The listing builds one solid part. Answer for the finished solid, in the listing's coordinates (mm). Face numbers are marked on the shaded views. A direction names the side the tool comes from. Give positions to 0.01 mm unless a question says otherwise; leave off trailing zeros. Write each loop counter-clockwise with the first axis right and the second up, starting at its lowest first coordinate (ties: lowest second). Pieces come first, ordered by that corner, then holes. Notation, with made-up numbers: (69, 54) - (106, 54) arc R31 cw to (106, 79) - close; hole circle Ø9 at (-18.5, -32.75). An arc over 180 degrees is marked (long way). One line per question, with ' | ' between items. Start each with the question number.
1. The mould has two halves that part along X. Classify the marked faces 5, 6, 7 and 8: +X half, -X half, draft (parallel to the pull), parting line (faces both ways), or undercut.
2. For the marked faces 1, 2, 3 and 4, determine the directions among +Z, -Z, +X, -X, +Y, -Y from which every point of the face is accessible in a straight line to the end or side of a thin tool.
3. A cutting plane is placed at A-A (z = 25). Determine the outline of the cut face in (x, y).
4. Given P1, Ø2, axis at y = 6.5, z = -7.5, coming from the -X side; P2, Ø10, axis at x = 1.5, y = 9.5, coming from the -Z side; P3, Ø10, axis at y = 6, z = -20.5, coming from the -X side; P4, Ø6, axis at x = -1.3, z = 25, coming from the -Y side, each flat-ended and moving along its own axis, determine where each tip first touches the part or whether it passes through.
5. A cutting plane is placed at D-D (z = 14.5). Determine the outline of the cut face in (x, y), then the cut area to 3 significant figures.
6. A cutting plane is placed at B-B (y = 14.5). Determine the outline of the cut face in (x, z), then the cut area to 3 significant figures.
7. Find the intervals of material crossed by L1, parallel to X at y = 9, z = 25; L2, parallel to X at y = 4.75, z = 37; L3, parallel to X at y = 12.25, z = -10, in increasing order. Write a range as from..to.
8. A cutting plane is placed at C-C (x = -13). Determine the outline of the cut face in (y, z).
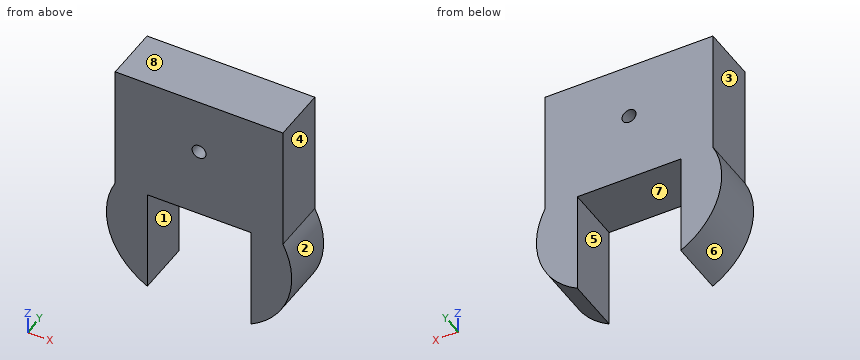
```python
from build123d import *

# Parameters (mm, degrees)
BOSS_EXTRUDE1_DEPTH = 20
SKETCH2_R           = 2.5
CUT_EXTRUDE1_DEPTH  = 20


with BuildPart() as part:
    # Sketch1 → Boss-Extrude1 (new body)
    with BuildSketch(Plane(origin=(0, 0, 0), x_dir=(1, 0, 0), z_dir=(0, 1, 0))):
        with BuildLine():
            Line((-19.801702617, 0), (17.198297383, 0))
            Line((17.198297383, 0), (17.198297383, 37))
            ThreePointArc((17.198297383, 37), (30.611248287, 20.881727984), (28.698297383, 0))
            Line((28.698297383, 0), (28.698297383, -45))
            Line((28.698297383, -45), (-31.301702617, -45))
            Line((-31.301702617, -45), (-31.301702617, 0))
            ThreePointArc((-31.301702617, 0), (-33.214653521, 20.881727984), (-19.801702617, 37))
            Line((-19.801702617, 37), (-19.801702617, 0))
        make_face()
    extrude(amount=BOSS_EXTRUDE1_DEPTH)

    # Sketch2 → Cut-Extrude1 (cut)
    with BuildSketch(Plane(origin=(0, 20, 0), x_dir=(1, 0, 0), z_dir=(0, 1, 0))):
        with Locations(Location((-1.301702617, -25, 0), (0, 0, 270))):
            Circle(SKETCH2_R)
    extrude(amount=-CUT_EXTRUDE1_DEPTH, mode=Mode.SUBTRACT)


solid = part.part
```
Determined:
1) face 5: undercut | face 6: -X half | face 7: undercut | face 8: draft
2) face 1: -Z, +Y, -Y | face 2: +X, +Y, -Y | face 3: +Z, -X, +Y, -Y | face 4: +Z, +X, +Y, -Y
3) outline: (-31.3, 0) - (-3.8, 0) - (-3.8, 20) - (-31.3, 20) - close; (1.2, 0) - (28.7, 0) - (28.7, 20) - (1.2, 20) - close
4) P1: x = -34.12 | P2: z = 0 | P3: x = -34.31 | P4: y = 0
5) outline: (-31.3, 0) - (28.7, 0) - (28.7, 20) - (-31.3, 20) - close | area: 1,200 mm2
6) outline: (-31.3, 0) arc R27.4 ccw to (-19.8, -37) - (-19.8, 0) - (17.2, 0) - (17.2, -37) arc R27.4 ccw to (28.7, 0) - (28.7, 45) - (-31.3, 45) - close; hole circle Ø5 at (-1.3, 25) | area: 3,530 mm2
7) L1: -31.3..-3.8, 1.2..28.7 | L2: -31.3..28.7 | L3: -34.31..-19.8, 17.2..31.71
8) outline: (0, 0) - (20, 0) - (20, 45) - (0, 45) - close
